Verification items for this drawing (mm, ordinates from the low corner). Give positions to 0.01 mm unless a question says otherwise; leave off trailing zeros. Order: outer loops, then holes, each group sorted by start corner. A loop starts at its lowest first (then second) coordinate and runs counter-clockwise, first axis right, second up.
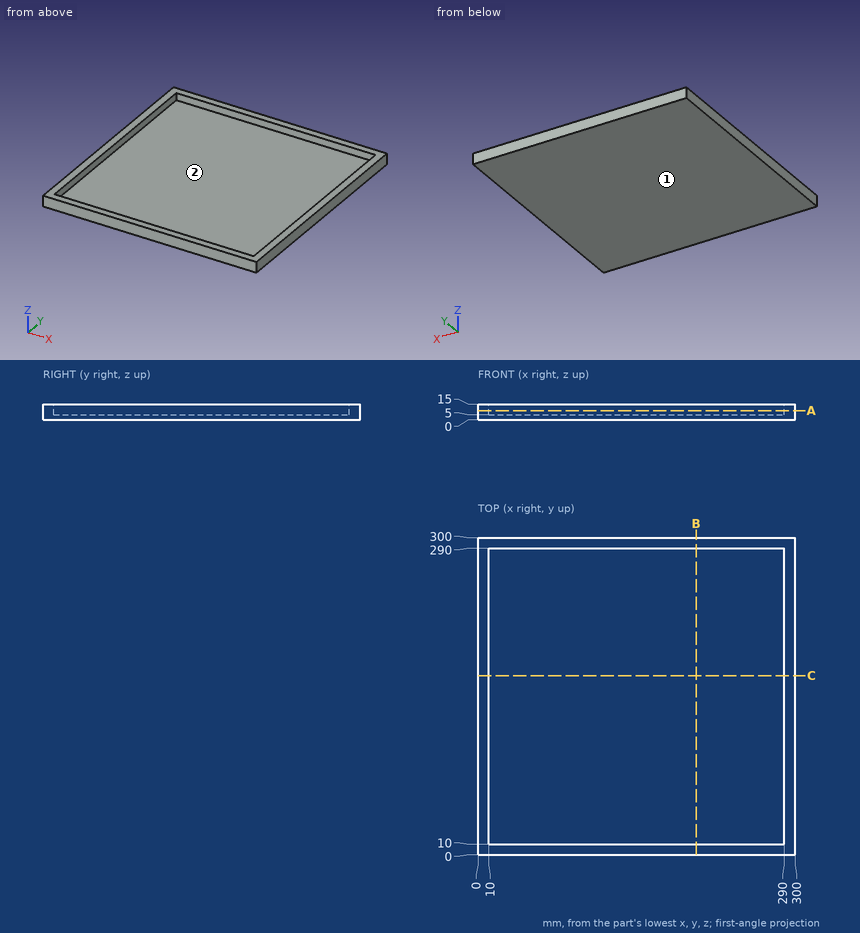
Q1. Thickness scan on L1, parallel to X at y = 78, z = 10.5; L2, parallel to Z at x = 288, y = 109.5. Record the ranges inside material, lowest first.
Q2. Cross-section at A-A, the plane z = 8.75. Record the boundary of the cut face in (x, y).
Q3. Cross-section at B-B, the plane x = 206.5. Record the boundary of the cut face in (y, z), and give its area (3 significant figures).
Q4. Gauge pin test, flat end, axial feed: P1, Ø10, axis at x = 141, y = 184, coming from the +Z side. Record the tip position at first contact, or that the pin passes through.
Q5. Release check for a two-part mould opening along Y. For the marked faces 1 and 2 record: pulls with the +Y half, pulls with the -Y half, needs draft (parallel to the pull), parting line crosses it, or undercut.
Answers follow:
1. L1: x = 0 to 10, 290 to 300
1. L2: z = 0 to 5
2. outline: (0, 0) - (300, 0) - (300, 300) - (0, 300) - close; hole (10, 10) - (290, 10) - (290, 290) - (10, 290) - close
3. outline: (0, 0) - (300, 0) - (300, 15) - (290, 15) - (290, 5) - (10, 5) - (10, 15) - (0, 15) - close
3. area: 1,700 mm2
4. P1: stops at z = 5
5. face 1: needs draft
5. face 2: undercut
